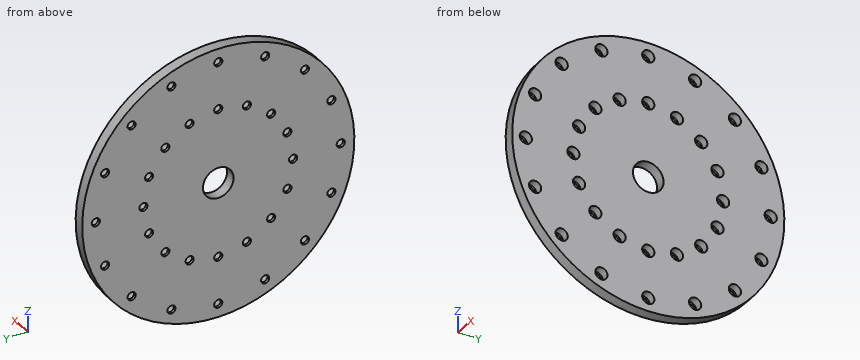
```python
from build123d import *

# Parameters (mm, degrees)
SKETCH1_R               = 200
BOSS_EXTRUDE1_DEPTH     = 16
CUT_EXTRUDE1_DEPTH      = 284.294899354
CUT_EXTRUDE1_DEPTH_BACK = 284.294899354
SKETCH2_R               = 22.5
SKETCH3_R               = 6
CUT_EXTRUDE2_DEPTH      = 284.294899354
CIRPATTERN1_COUNT       = 16
SKETCH4_R               = 6
CUT_EXTRUDE3_DEPTH      = 284.294899354
CIRPATTERN2_COUNT       = 16
SKETCH5_R               = 9
CUT_EXTRUDE4_DEPTH      = 12
CIRPATTERN3_COUNT       = 16
SKETCH6_R               = 9
CUT_EXTRUDE5_DEPTH      = 12
CIRPATTERN4_COUNT       = 16


with BuildPart() as part:
    # Sketch1 → Boss-Extrude1 (new body)
    with BuildSketch(Plane(origin=(0, 0, 0), x_dir=(0, 0, -1), z_dir=(1, 0, 0))):
        Circle(SKETCH1_R)
    extrude(amount=BOSS_EXTRUDE1_DEPTH)

    # Sketch2 → Cut-Extrude1 (cut, two sides: drawn at the far end of the back side and taken through both)
    with BuildSketch(Plane(origin=(16, 0, 0), x_dir=(0, 0, -1), z_dir=(1, 0, 0)).offset(-CUT_EXTRUDE1_DEPTH_BACK)):
        Circle(SKETCH2_R)
    extrude(amount=CUT_EXTRUDE1_DEPTH + CUT_EXTRUDE1_DEPTH_BACK, mode=Mode.SUBTRACT)

    # Sketch3 → Cut-Extrude2 (cut, symmetric)
    with BuildSketch(Plane(origin=(16, 0, 0), x_dir=(0, 0, -1), z_dir=(1, 0, 0))):
        with Locations((110, 0)):
            Circle(SKETCH3_R)
    cut_extrude2 = extrude(amount=CUT_EXTRUDE2_DEPTH, both=True, mode=Mode.SUBTRACT)

    # CirPattern1: Cut-Extrude2 ×16 about axis
    cirpattern1_axis = Axis((0, 0, 0), (1, 0, 0))
    for i in range(1, CIRPATTERN1_COUNT):
        add(cut_extrude2.rotate(cirpattern1_axis, i * 360 / CIRPATTERN1_COUNT), mode=Mode.SUBTRACT)

    # Sketch4 → Cut-Extrude3 (cut, symmetric)
    with BuildSketch(Plane(origin=(16, 0, 0), x_dir=(0, 0, -1), z_dir=(1, 0, 0))):
        with Locations((180, 0)):
            Circle(SKETCH4_R)
    cut_extrude3 = extrude(amount=CUT_EXTRUDE3_DEPTH, both=True, mode=Mode.SUBTRACT)

    # CirPattern2: Cut-Extrude3 ×16 about axis
    cirpattern2_axis = Axis((0, 0, 0), (1, 0, 0))
    for i in range(1, CIRPATTERN2_COUNT):
        add(cut_extrude3.rotate(cirpattern2_axis, i * 360 / CIRPATTERN2_COUNT), mode=Mode.SUBTRACT)

    # Sketch5 → Cut-Extrude4 (cut)
    with BuildSketch(Plane(origin=(16, 0, 0), x_dir=(0, 0, -1), z_dir=(1, 0, 0))):
        with Locations((166.298315852, 68.883017826)):
            Circle(SKETCH5_R)
    cut_extrude4 = extrude(amount=-CUT_EXTRUDE4_DEPTH, mode=Mode.SUBTRACT)

    # CirPattern3: Cut-Extrude4 ×16 about axis
    cirpattern3_axis = Axis((0, 0, 0), (1, 0, 0))
    for i in range(1, CIRPATTERN3_COUNT):
        add(cut_extrude4.rotate(cirpattern3_axis, i * 360 / CIRPATTERN3_COUNT), mode=Mode.SUBTRACT)

    # Sketch6 → Cut-Extrude5 (cut)
    with BuildSketch(Plane(origin=(16, 0, 0), x_dir=(0, 0, -1), z_dir=(1, 0, 0))):
        with Locations((101.626748576, 42.09517756)):
            Circle(SKETCH6_R)
    cut_extrude5 = extrude(amount=-CUT_EXTRUDE5_DEPTH, mode=Mode.SUBTRACT)

    # CirPattern4: Cut-Extrude5 ×16 about axis
    cirpattern4_axis = Axis((0, 0, 0), (1, 0, 0))
    for i in range(1, CIRPATTERN4_COUNT):
        add(cut_extrude5.rotate(cirpattern4_axis, i * 360 / CIRPATTERN4_COUNT), mode=Mode.SUBTRACT)


solid = part.part
```
Model file for the job. Use its own axes, mm. Give positions to 0.01 mm unless a question says otherwise; leave off trailing zeros. Order: outer loops, then holes, each group sorted by start corner. A loop starts at its lowest first (then second) coordinate and runs counter-clockwise, first axis right, second up.
1) Saw through at C-C, the plane x = 13.25. Count the separate pieces of the cut face and the enclosed holes in it, then the cut area to 3 significant figures.
2) Wall check: probe 1 along Y at (x, z) = (7.5, 0); probe 2 along Y at (x, z) = (12.5, 131.5); probe 3 along Y at (x, z) = (4.5, 162.5). Give the ranges that are in metal, low to high.
3) Pin check, flat tips, straight feed: pin 1 (5.5 mm diameter, centred on y = -3, z = 111.5, fed in from +X); pin 2 (1 mm diameter, centred on x = 3.5, y = -139, fed in from +Z); pin 3 (11 mm diameter, centred on y = 0, z = 110, fed in from -X); pin 4 (5 mm diameter, centred on x = 2.5, z = 22.5, fed in from +Y). Stop position of each tip, or through.
4) Saw through at A-A, the plane y = 180. Write the cut outline in (x, z), then the cut area to 3 significant figures.
Computed:
1. separate pieces: 1
1. enclosed holes: 33
1. area: 116,000 mm2
2. probe 1: y = -200 to -189, -171 to -119, -101 to -22.5, 22.5 to 101, 119 to 171, 189 to 200
2. probe 2: y = -150.69 to -135.23, -119.33 to 119.33, 135.23 to 150.69
2. probe 3: y = -116.59 to -77.04, -60.72 to 60.72, 77.04 to 116.59
3. pin 1: stops at x = 4
3. pin 2: stops at z = 144.28
3. pin 3: passes through
3. pin 4: stops at y = 199
4. outline: (0, -87.18) - (16, -87.18) - (16, -9) - (4, -9) - (4, -6) - (0, -6) - close; (0, 6) - (4, 6) - (4, 9) - (16, 9) - (16, 87.18) - (0, 87.18) - close
4. area: 2,530 mm2
